```python
from build123d import *

# Parameters (mm, degrees)
BOSS_EXTRUDE4_DEPTH             = 154
BOSS_EXTRUDE5_REACH             = 216.516
SKETCH11_W                      = 4
SKETCH11_H                      = 7
BOSS_EXTRUDE5_DIRECTION_2_REACH = 216.516
BOSS_EXTRUDE6_DEPTH             = 45
SKETCH15_W                      = 138
SKETCH15_H                      = 4
SKETCH15_W_2                    = 154
BOSS_EXTRUDE7_DEPTH             = 8
SKETCH16_W                      = 150
SKETCH16_H                      = 3
SKETCH16_W_2                    = 142
SKETCH16_H_2                    = 4
BOSS_EXTRUDE8_DEPTH             = 8
CUT_EXTRUDE2_DEPTH              = 229.781555201
CUT_EXTRUDE2_DEPTH_BACK         = 229.781555201
SKETCH19_R                      = 12
SKETCH19_R_2                    = 1.25
CUT_EXTRUDE3_REACH              = 184.047
FILLET3_R                       = 2


with BuildPart() as part:
    # Sketch3 → Boss-Extrude4 (new body)
    with BuildSketch(Plane.XY):
        Polygon((-80, 0), (80, 0), (80, 10), (69, 10), (69, 6), (77, 6), (77, 3), (-77, 3), (-77, 6), (-69, 6), (-69, 10), (-80, 10), align=None)
    extrude(amount=BOSS_EXTRUDE4_DEPTH)

    # Sketch11 → Boss-Extrude5 (add, up to next)
    with BuildSketch(Plane(origin=(-69, 0, 0), x_dir=(0, 0, -1), z_dir=(1, 0, 0)), mode=Mode.PRIVATE) as boss_extrude5_sk1:
        with Locations((-152, 6.5)):
            Rectangle(SKETCH11_W, SKETCH11_H)
    boss_extrude5_tool1 = extrude(boss_extrude5_sk1.sketch, amount=BOSS_EXTRUDE5_REACH, mode=Mode.PRIVATE) - part.part
    add(boss_extrude5_tool1.solids().sort_by_distance((-69, 6.5, 152))[0])

    # Sketch11 → Boss-Extrude5 direction 2 (add, up to next)
    with BuildSketch(Plane(origin=(-69, 0, 0), x_dir=(0, 0, -1), z_dir=(1, 0, 0)), mode=Mode.PRIVATE) as boss_extrude5_direction_2_sk1:
        with Locations((-152, 6.5)):
            Rectangle(SKETCH11_W, SKETCH11_H)
    boss_extrude5_direction_2_tool1 = extrude(boss_extrude5_direction_2_sk1.sketch, amount=-BOSS_EXTRUDE5_DIRECTION_2_REACH, mode=Mode.PRIVATE) - part.part
    add(boss_extrude5_direction_2_tool1.solids().sort_by_distance((-69, 6.5, 152))[0])

    # Sketch13 → Boss-Extrude6 (add)
    with BuildSketch(Plane(origin=(0, 10, 0), x_dir=(1, 0, 0), z_dir=(0, 1, 0))):
        Polygon((80, 0), (77, 0), (77, -150), (-77, -150), (-77, 0), (-80, 0), (-80, -154), (80, -154), align=None)
    extrude(amount=BOSS_EXTRUDE6_DEPTH)

    # Sketch15 → Boss-Extrude7 (add)
    with BuildSketch(Plane(origin=(0, 0, 150), x_dir=(-1, 0, 0), z_dir=(0, 0, -1))):
        with Locations((0, 8)):
            Rectangle(SKETCH15_W, SKETCH15_H)
        with Locations((0, 15)):
            Rectangle(SKETCH15_W_2, SKETCH15_H)
    extrude(amount=BOSS_EXTRUDE7_DEPTH)

    # Sketch16 → Boss-Extrude8 (add)
    with BuildSketch(Plane(origin=(-77, 0, 0), x_dir=(0, 0, -1), z_dir=(1, 0, 0))):
        with Locations((-75, 46.5)):
            Rectangle(SKETCH16_W, SKETCH16_H)
        with Locations((-71, 15)):
            Rectangle(SKETCH16_W_2, SKETCH16_H_2)
        with Locations((-75, 53)):
            Rectangle(SKETCH16_W, SKETCH16_H_2)
    boss_extrude8 = extrude(amount=BOSS_EXTRUDE8_DEPTH)

    # Mirror1: Boss-Extrude8 across plane
    add(boss_extrude8.mirror(Plane(origin=(0, 0, 0), x_dir=(0, 0, 1), z_dir=(1, 0, 0))))

    # Sketch19 → Cut-Extrude2 (cut, two sides: drawn at the far end of the back side and taken through both)
    with BuildSketch(Plane(origin=(80, 0, 0), x_dir=(0, 0, -1), z_dir=(1, 0, 0)).offset(-CUT_EXTRUDE2_DEPTH_BACK)):
        with Locations(Location((-77, 31, 0), (0, 0, 180))):
            Circle(SKETCH19_R)
        with Locations(Location((-58, 31, 0), (0, 0, 180))):
            Circle(SKETCH19_R_2)
        with Locations(Location((-96, 31, 0), (0, 0, 180))):
            Circle(SKETCH19_R_2)
    extrude(amount=CUT_EXTRUDE2_DEPTH + CUT_EXTRUDE2_DEPTH_BACK, mode=Mode.SUBTRACT)

    # Sketch27 → Cut-Extrude3 (cut, up to next)
    with BuildSketch(Plane.XZ, mode=Mode.PRIVATE) as cut_extrude3_sk1:
        Polygon((-57.47846256, 25.321688373), (-24.93570827, 25.321688373), (-19.305381247, 29.819289123), (-24.499608086, 36.321688373), (-54.771412112, 36.321688373), (-61.574151377, 29.276341528), align=None)
    cut_extrude3_tool1 = extrude(cut_extrude3_sk1.sketch, amount=-CUT_EXTRUDE3_REACH, mode=Mode.PRIVATE) & part.part
    # Sketch27 → Cut-Extrude3 (cut, up to next)
    with BuildSketch(Plane.XZ, mode=Mode.PRIVATE) as cut_extrude3_sk2:
        Polygon((-56.617071459, 38.369250276), (-63.55245833, 31.186525183), (-68.252983819, 35.725187368), (-61.359608852, 74.819459497), (-51.28413594, 68.613830533), align=None)
    cut_extrude3_tool2 = extrude(cut_extrude3_sk2.sketch, amount=-CUT_EXTRUDE3_REACH, mode=Mode.PRIVATE) & part.part
    # Sketch27 → Cut-Extrude3 (cut, up to next)
    with BuildSketch(Plane.XZ, mode=Mode.PRIVATE) as cut_extrude3_sk3:
        Polygon((-22.615548373, 38.369250276), (-17.156752628, 31.535650116), (-11.912075272, 35.725187368), (-5.018700304, 74.819459497), (-17.282612854, 68.613830533), align=None)
    cut_extrude3_tool3 = extrude(cut_extrude3_sk3.sketch, amount=-CUT_EXTRUDE3_REACH, mode=Mode.PRIVATE) & part.part
    # Sketch27 → Cut-Extrude3 (cut, up to next)
    with BuildSketch(Plane.XZ, mode=Mode.PRIVATE) as cut_extrude3_sk4:
        Polygon((-57.266645874, 77), (-49.434486563, 72.176060211), (-17.400076182, 72.176060211), (-7.866735395, 77), (-15.460479394, 83.176060211), (-47.494889775, 83.176060211), align=None)
    cut_extrude3_tool4 = extrude(cut_extrude3_sk4.sketch, amount=-CUT_EXTRUDE3_REACH, mode=Mode.PRIVATE) & part.part
    # Sketch27 → Cut-Extrude3 (cut, up to next)
    with BuildSketch(Plane.XZ, mode=Mode.PRIVATE) as cut_extrude3_sk5:
        Polygon((-60.734283515, 78.365855711), (-53.840908548, 117.46012784), (-47.581510302, 123.087083774), (-42.646926869, 117.59787731), (-48.163667933, 86.310884009), align=None)
    cut_extrude3_tool5 = extrude(cut_extrude3_sk5.sketch, amount=-CUT_EXTRUDE3_REACH, mode=Mode.PRIVATE) & part.part
    # Sketch27 → Cut-Extrude3 (cut, up to next)
    with BuildSketch(Plane.XZ, mode=Mode.PRIVATE) as cut_extrude3_sk6:
        Polygon((-14.162144847, 86.310884009), (-4.393374967, 78.365855711), (2.5, 117.46012784), (-2.235185266, 123.038840685), (-8.645403783, 117.59787731), align=None)
    cut_extrude3_tool6 = extrude(cut_extrude3_sk6.sketch, amount=-CUT_EXTRUDE3_REACH, mode=Mode.PRIVATE) & part.part
    # Sketch27 → Cut-Extrude3 (cut, up to next)
    with BuildSketch(Plane.XZ, mode=Mode.PRIVATE) as cut_extrude3_sk7:
        Polygon((-45.536395336, 124.925562704), (-41.444496972, 120.373754987), (-9.624660978, 120.373754987), (-4.014751663, 125.13541967), (-9.309821385, 131.373754987), (-38.363457794, 131.373754987), align=None)
    cut_extrude3_tool7 = extrude(cut_extrude3_sk7.sketch, amount=-CUT_EXTRUDE3_REACH, mode=Mode.PRIVATE) & part.part
    # Sketch27 → Cut-Extrude3 (cut, up to next)
    with BuildSketch(Plane.XZ, mode=Mode.PRIVATE) as cut_extrude3_sk8:
        Polygon((8.274521259, 25.321688373), (40.817275549, 25.321688373), (46.447602573, 29.819289123), (41.253375733, 36.321688373), (10.981571707, 36.321688373), (4.178832443, 29.276341528), align=None)
    cut_extrude3_tool8 = extrude(cut_extrude3_sk8.sketch, amount=-CUT_EXTRUDE3_REACH, mode=Mode.PRIVATE) & part.part
    # Sketch27 → Cut-Extrude3 (cut, up to next)
    with BuildSketch(Plane.XZ, mode=Mode.PRIVATE) as cut_extrude3_sk9:
        Polygon((9.13591236, 38.369250276), (2.200525489, 31.186525183), (-2.5, 35.725187368), (4.393374967, 74.819459497), (14.46884788, 68.613830533), align=None)
    cut_extrude3_tool9 = extrude(cut_extrude3_sk9.sketch, amount=-CUT_EXTRUDE3_REACH, mode=Mode.PRIVATE) & part.part
    # Sketch27 → Cut-Extrude3 (cut, up to next)
    with BuildSketch(Plane.XZ, mode=Mode.PRIVATE) as cut_extrude3_sk10:
        Polygon((43.137435446, 38.369250276), (48.596231191, 31.535650116), (53.840908548, 35.725187368), (60.734283515, 74.819459497), (48.470370966, 68.613830533), align=None)
    cut_extrude3_tool10 = extrude(cut_extrude3_sk10.sketch, amount=-CUT_EXTRUDE3_REACH, mode=Mode.PRIVATE) & part.part
    # Sketch27 → Cut-Extrude3 (cut, up to next)
    with BuildSketch(Plane.XZ, mode=Mode.PRIVATE) as cut_extrude3_sk11:
        Polygon((8.486337945, 77), (16.318497257, 72.176060211), (48.352907637, 72.176060211), (57.886248425, 77), (50.292504425, 83.176060211), (18.258094045, 83.176060211), align=None)
    cut_extrude3_tool11 = extrude(cut_extrude3_sk11.sketch, amount=-CUT_EXTRUDE3_REACH, mode=Mode.PRIVATE) & part.part
    # Sketch27 → Cut-Extrude3 (cut, up to next)
    with BuildSketch(Plane.XZ, mode=Mode.PRIVATE) as cut_extrude3_sk12:
        Polygon((5.018700304, 78.365855711), (11.912075272, 117.46012784), (18.171473518, 123.087083774), (23.106056951, 117.59787731), (17.589315886, 86.310884009), align=None)
    cut_extrude3_tool12 = extrude(cut_extrude3_sk12.sketch, amount=-CUT_EXTRUDE3_REACH, mode=Mode.PRIVATE) & part.part
    # Sketch27 → Cut-Extrude3 (cut, up to next)
    with BuildSketch(Plane.XZ, mode=Mode.PRIVATE) as cut_extrude3_sk13:
        Polygon((51.590838973, 86.310884009), (61.359608852, 78.365855711), (68.252983819, 117.46012784), (63.517798554, 123.038840685), (57.107580037, 117.59787731), align=None)
    cut_extrude3_tool13 = extrude(cut_extrude3_sk13.sketch, amount=-CUT_EXTRUDE3_REACH, mode=Mode.PRIVATE) & part.part
    # Sketch27 → Cut-Extrude3 (cut, up to next)
    with BuildSketch(Plane.XZ, mode=Mode.PRIVATE) as cut_extrude3_sk14:
        Polygon((20.216588483, 124.925562704), (24.308486848, 120.373754987), (56.128322842, 120.373754987), (61.738232157, 125.13541967), (56.443162434, 131.373754987), (27.389526025, 131.373754987), align=None)
    cut_extrude3_tool14 = extrude(cut_extrude3_sk14.sketch, amount=-CUT_EXTRUDE3_REACH, mode=Mode.PRIVATE) & part.part
    add(cut_extrude3_tool1.solids().sort_by_distance((-40.338799, 0, 30.704471))[0], mode=Mode.SUBTRACT)
    add(cut_extrude3_tool2.solids().sort_by_distance((-59.857835, 0, 52.918339))[0], mode=Mode.SUBTRACT)
    add(cut_extrude3_tool3.solids().sort_by_distance((-14.193031, 0, 53.066237))[0], mode=Mode.SUBTRACT)
    add(cut_extrude3_tool4.solids().sort_by_distance((-32.455956, 0, 77.628005))[0], mode=Mode.SUBTRACT)
    add(cut_extrude3_tool5.solids().sort_by_distance((-51.306641, 0, 101.288791))[0], mode=Mode.SUBTRACT)
    add(cut_extrude3_tool6.solids().sort_by_distance((-5.750482, 0, 101.274794))[0], mode=Mode.SUBTRACT)
    add(cut_extrude3_tool7.solids().sort_by_distance((-24.675646, 0, 125.760601))[0], mode=Mode.SUBTRACT)
    add(cut_extrude3_tool8.solids().sort_by_distance((25.414185, 0, 30.704471))[0], mode=Mode.SUBTRACT)
    add(cut_extrude3_tool9.solids().sort_by_distance((5.895149, 0, 52.918339))[0], mode=Mode.SUBTRACT)
    add(cut_extrude3_tool10.solids().sort_by_distance((51.559953, 0, 53.066237))[0], mode=Mode.SUBTRACT)
    add(cut_extrude3_tool11.solids().sort_by_distance((33.297027, 0, 77.628005))[0], mode=Mode.SUBTRACT)
    add(cut_extrude3_tool12.solids().sort_by_distance((14.446343, 0, 101.288791))[0], mode=Mode.SUBTRACT)
    add(cut_extrude3_tool13.solids().sort_by_distance((60.002501, 0, 101.274794))[0], mode=Mode.SUBTRACT)
    add(cut_extrude3_tool14.solids().sort_by_distance((41.077338, 0, 125.760601))[0], mode=Mode.SUBTRACT)

    # Fillet3
    fillet3_edges = [part.edges().sort_by_distance(p)[0] for p in [
        (-80, 0, 77),
        (80, 0, 77),
        (80, 55, 77),
        (-80, 55, 77),
    ]]
    fillet(fillet3_edges, radius=FILLET3_R)


solid = part.part
```
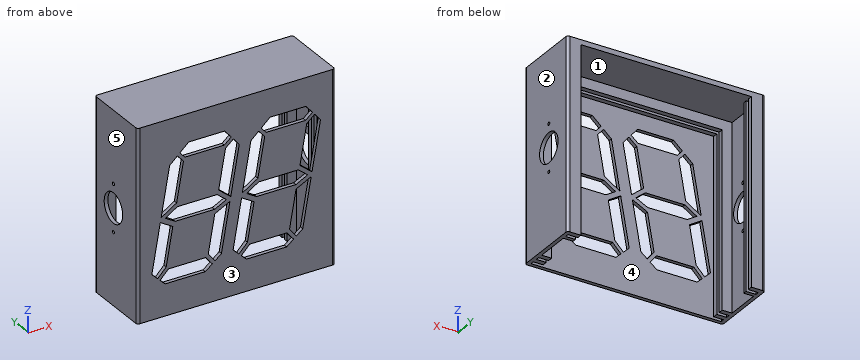
Source: CAD feature listing. Evaluate the final solid. Frame: model axes, mm. Face numbers are marked on the shaded views. A direction names the side the tool comes from. Round coordinates to 2 decimals unless told otherwise and drop trailing zeros. Write each loop counter-clockwise with the first axis right and the second up, starting at its lowest first coordinate (ties: lowest second). Pieces come first, ordered by that corner, then holes. Notation, with made-up numbers: M -18.75,53 L 37.25,53 A23 cw 37.25,83 Z; hole C 20,62 d9. An arc over 180 degrees is marked long. Answer as a JSON object with one key per item and string values. Group by question number.
(1) Section query B-B on z = 61.5. State how many separate pieces and enclosed holes the cut face has, then the cut area to 3 significant figures.
(2) Mould query, pull axis X, two halves, no side actions, for the marked faces 1, 2 and 3. Classes: +X half, -X half, draft (parallel to the pull), parting line (faces both ways), or undercut.
(3) Section query A-A on y = 40. Output: boundary loops of the cut face in (x, z), then the cut area to 3 significant figures.
(4) Ray query, line 1 (X direction, y = 5, z = 61); line 2 (Y direction, x = -78, z = 77); line 3 (X direction, y = 8, z = 109.5). Return the intervals inside material, ascending. Write a range as [from, to].
(5) Reachability of the marked faces 4 and 5 from +Z, -Z, +X, -X, +Y, -Y: full face, straight path, thin tool, end or side. Return the list, or none.
(6) First-contact query: pin 1 (1.2 mm diameter, centred on x = 18.5, y = 7.5, fed in from -Z); pin 2 (6 mm diameter, centred on x = -11.5, z = 95, fed in from +Y); pin 3 (4 mm diameter, centred on x = -9, y = 24, fed in from -Z). Flat tips, straight axial feed; report the tip coordinate or a pass-through.
Computed values:
{
 "1": {"separate pieces": "5", "enclosed holes": "0", "area": "895 mm^2"},
 "2": {"face 1": "undercut", "face 2": "+X half", "face 3": "draft"},
 "3": {"outline": "M -80,0 L -77,0 L -77,69.06 L -80,69.06 Z; M -80,84.94 L -77,84.94 L -77,150 L 77,150 L 77,84.94 L 80,84.94 L 80,154 L -80,154 Z; M 77,0 L 80,0 L 80,69.06 L 77,69.06 Z", "area": "1,440 mm^2"},
 "4": {"line 1": "[-80, -77], [77, 80]", "line 2": "[0, 19], [43, 55]", "line 3": "[-80, -69], [69, 80]"},
 "5": {"face 4": "-Z", "face 5": "+Z, -Z, -X, +Y, -Y"},
 "6": {"pin 1": "z = 142", "pin 2": "y = 3", "pin 3": "z = 150"}
}
